Work out the finished part from the listing and answer in its coordinate system (mm). A direction names the side the tool comes from. Round coordinates to 2 decimals unless told otherwise and drop trailing zeros. Write each loop counter-clockwise with the first axis right and the second up, starting at its lowest first coordinate (ties: lowest second). Pieces come first, ordered by that corner, then holes. Notation, with made-up numbers: (35.25, 27) -> (81.25, 27) arc R30 ccw to (81.25, 51) -> close; hole circle Ø6 at (72, 14). An arc over 180 degrees is marked (long way). One line per item, written item: value.
```python
from build123d import *

# Parameters (mm, degrees)
F0_W     = 5.5
F0_H     = 5
F0_W_2   = 7.5
F0_H_2   = 6
F1_DEPTH = 40
F2_R     = 5
F3_R     = 13.75
F4_DEPTH = 25


with BuildPart() as f1:
    # F0 (on Front) → F1 (new body)
    with BuildSketch(Plane.XZ):
        Polygon((0, 72), (0, 0), (6, 0), (6, 66), (6, 72), align=None)
        Polygon((6, 72), (6, 66), (13.5, 66), (19, 66), (19, 72), align=None)
        with Locations((16.25, 63.5)):
            Rectangle(F0_W, F0_H)
        with Locations((22.75, 69)):
            Rectangle(F0_W_2, F0_H_2)
        Polygon((32.5, 72), (26.5, 72), (26.5, 66), (26.5, 47), (32.5, 47), align=None)
    extrude(amount=F1_DEPTH)

    # F2
    f2_edges = [f1.edges().sort_by_distance(p)[0] for p in [
        (3, 0, 0),
        (3, -40, 0),
    ]]
    fillet(f2_edges, radius=F2_R)

    # F3 (on face) → F4 (cut)
    with BuildSketch(Plane(origin=(0, 0, 0), x_dir=(0, -1, 0), z_dir=(-1, 0, 0))):
        with Locations((20, 20)):
            Circle(F3_R)
    extrude(amount=-F4_DEPTH, mode=Mode.SUBTRACT)


solid = f1.part
```
(1) Consider probe 1 along X at (y, z) = (-17, 48); probe 2 along Z at (x, y) = (2.4, -20); probe 3 along X at (y, z) = (-6, 25). Determine where each line is inside the solid, lowest interval first.
Reported:
probe 1: x = 0 to 6, 26.5 to 32.5
probe 2: z = 0 to 6.25, 33.75 to 72
probe 3: x = 0 to 6
(2) Flat-ended cylindrical pins translate along their axes: pin 1 Ø1.5 at (x, y) = (24.5, -31.5) entering from -Z; pin 2 Ø6 at (x, y) = (17.5, -26) entering from -Z; pin 3 Ø1.8 at (x, y) = (28.5, -18.5) entering from -Z. Find the tip coordinate at first contact, or state that the pin passes through.
Reported:
pin 1: stops at z = 66
pin 2: stops at z = 61
pin 3: stops at z = 47
(3) Find section D-D on y = -11. Give the vertices of the cut face in (x, z).
Reported:
outline: (0, 0) -> (6, 0) -> (6, 9.6) -> (0, 9.6) -> close; (0, 30.4) -> (6, 30.4) -> (6, 66) -> (13.5, 66) -> (13.5, 61) -> (19, 61) -> (19, 66) -> (26.5, 66) -> (26.5, 47) -> (32.5, 47) -> (32.5, 72) -> (0, 72) -> close
(4) Find section C-C on x = 15.5. Give the vertices of the cut face in (y, z).
Reported:
outline: (-40, 61) -> (0, 61) -> (0, 72) -> (-40, 72) -> close
(5) Find section A-A on y = -20. Give the vertices of the cut face in (x, z), plus the area to 4 significant figures.
Reported:
outline: (0, 0) -> (6, 0) -> (6, 6.25) -> (0, 6.25) -> close; (0, 33.75) -> (6, 33.75) -> (6, 66) -> (13.5, 66) -> (13.5, 61) -> (19, 61) -> (19, 66) -> (26.5, 66) -> (26.5, 47) -> (32.5, 47) -> (32.5, 72) -> (0, 72) -> close
area: 567.5 mm2
(6) A tool of negligible diameter and unlimited length cuts with its end or side. For faces 1 (the face through (16, -20, 61)), 2 (the face through (29, -20, 47)), 3 (the face through (3, -38, 1)), from which of +Z, -Z, +X, -X, +Y, -Y can it reach the whole face along a straight path? Write none if from no direction.
Reported:
face 1: -Z, +Y, -Y
face 2: -Z, +X, +Y, -Y
face 3: -Z, +X, -X, -Y
(7) Find section B-B on z = 20. Give the vertices of the cut face in (x, y).
Reported:
outline: (0, -40) -> (6, -40) -> (6, -33.75) -> (0, -33.75) -> close; (0, -6.25) -> (6, -6.25) -> (6, 0) -> (0, 0) -> close
(8) For a pull along Z with two mould halves and no side action, classify faces 4 (the face through (0, -20, 45)), 5 (the face through (2.958, -33.115, 24.13)), 6 (the face through (23, -20, 66)) as pulls with the +Z half, pulls with the -Z half, needs draft (parallel to the pull), parting line crosses it, or undercut.
Reported:
face 4: needs draft
face 5: undercut
face 6: pulls with the -Z half
